```python
from build123d import *

# Parameters (mm, degrees)
CUT_EXTRUDE1_DEPTH = 2.5


with BuildPart() as part:
    # Sketch1 → Revolve1 (revolve)
    with BuildSketch(Plane.XY):
        Polygon((0, 2.5), (0, 4.25), (-4.5, 4.25), (-5, 3.75), (-5, 0), (16, 0), (16, 2.067), (15.567, 2.5), align=None)
    revolve(axis=Axis((16, 0, 0), (-1, 0, 0)))

    # Sketch2 → Cut-Extrude1 (cut)
    with BuildSketch(Plane.ZY.offset(5)):
        Polygon((0, 2.309401077), (-2, 1.154700538), (-2, -1.154700538), (0, -2.309401077), (2, -1.154700538), (2, 1.154700538), align=None)
    extrude(amount=-CUT_EXTRUDE1_DEPTH, mode=Mode.SUBTRACT)


solid = part.part
```
Source: CAD feature listing. Evaluate the final solid. Frame: model axes, mm. A direction names the side the tool comes from. Give positions to 0.01 mm unless a question says otherwise; leave off trailing zeros. Loops run counter-clockwise (first coordinate to the right, second up) from the corner with the lowest first, then second, coordinate; pieces in that order, holes last. Notation, with made-up numbers: (78, -18.75) -> (123, -18.75) arc R12 cw to (123, -1.75) -> close; hole circle Ø11 at (0, 20). An arc over 180 degrees is marked (long way). Put each result on its own line as item: value. Start each with the question number.
1) Reachability of faces 4 (the face through (-3.768, 1.724, 1.014)), 5 (the face through (16, 0, 0)), 6 (the face through (7.67, -0.54, 2.44)) from +Z, -Z, +X, -X, +Y, -Y: full face, straight path, thin tool, end or side. Return the list, or none.
2) Material intervals for probe 1 along Y at (x, z) = (2.5, 1.5); probe 2 along X at (y, z) = (-1, -0.5), sorted ascending.
3) Draft query along Z for faces 1 (the face through (0, -2, 2)), 2 (the face through (-4, 0, -2)), 3 (the face through (-2.282, 2.285, -3.584)). Return one class per face: released by +Z, released by -Z, zero draft, split by the parting line, or undercut.
4) Cut plane C-C (x = 5.75). Return loops of the section in (y, z).
5) Cut plane A-A (y = 0). Return loops of the section in (x, z).
6) Cut plane B-B (x = -0.5). Return loops of the section in (y, z).
7) Contact query for flat-ended pins moving along their axis: P1, Ø3, axis at y = -0.5, z = 0, coming from the -X side; P2, Ø2, axis at x = 0, z = -2.5, coming from the -Y side; P3, Ø4, axis at x = 1, y = 2.5, coming from the +Z side. Output: stop coordinate, or through.
Results are:
1. face 4: -X
1. face 5: +Z, -Z, +X, +Y, -Y
1. face 6: +X
2. probe 1: y = -2 to 2
2. probe 2: x = -2.5 to 16
3. face 1: zero draft
3. face 2: undercut
3. face 3: split by the parting line
4. outline: circle Ø5 at (0, 0)
5. outline: (-5, -3.75) -> (-4.5, -4.25) -> (0, -4.25) -> (0, -2.5) -> (15.57, -2.5) -> (16, -2.07) -> (16, 2.07) -> (15.57, 2.5) -> (0, 2.5) -> (0, 4.25) -> (-4.5, 4.25) -> (-5, 3.75) -> (-5, 2) -> (-2.5, 2) -> (-2.5, -2) -> (-5, -2) -> close
6. outline: circle Ø8.5 at (0, 0)
7. P1: stops at x = -2.5
7. P2: stops at y = -3.98
7. P3: stops at z = 4.18
